```python
from build123d import *

# Parameters (mm, degrees)
SKETCH1_R           = 2.6
BOSS_EXTRUDE1_DEPTH = 20
BOSS_EXTRUDE2_DEPTH = 20
BOSS_EXTRUDE3_DEPTH = 180
CUT_EXTRUDE1_DEPTH  = 195.584574731


with BuildPart() as part:
    # Sketch1 → Boss-Extrude1 (new body)
    with BuildSketch(Plane(origin=(0, 0, 0), x_dir=(1, 0, 0), z_dir=(0, 1, 0))):
        with BuildLine():
            Line((10, 0), (-10, 0))
            ThreePointArc((-10, 0), (-2.947752983, 31.810630591), (16.887506811, 57.660444431))
            Line((16.887506811, 57.660444431), (29.743259005, 42.339555569))
            ThreePointArc((29.743259005, 42.339555569), (15.178402758, 23.358265357), (10, 0))
        make_face()
        with Locations(Location((0.770593323, 10, 0), (0, 0, 270))):
            Circle(SKETCH1_R, mode=Mode.SUBTRACT)
        with Locations(Location((6.115324888, 27.584447974, 0), (0, 0, 270))):
            Circle(SKETCH1_R, mode=Mode.SUBTRACT)
        with Locations(Location((16.150266317, 42.98181517, 0), (0, 0, 270))):
            Circle(SKETCH1_R, mode=Mode.SUBTRACT)
    extrude(amount=BOSS_EXTRUDE1_DEPTH)

    # Sketch2 → Boss-Extrude2 (add)
    with BuildSketch(Plane(origin=(0, 20, 0), x_dir=(1, 0, 0), z_dir=(0, 1, 0))):
        Polygon((16.887506811, 57.660444431), (29.743259005, 42.339555569), (34.416130108, 46.260559988), (21.560377914, 61.58144885), align=None)
    extrude(amount=-BOSS_EXTRUDE2_DEPTH)

    # Sketch4 → Cut-Extrude1 (cut, through all)
    with BuildSketch(Plane(origin=(0, 20, 0), x_dir=(1, 0, 0), z_dir=(0, 1, 0))):
        with BuildLine():
            Line((29.743259005, 42.339555569), (34.416130108, 46.260559988))
            Line((34.416130108, 46.260559988), (21.560377914, 61.58144885))
            Line((21.560377914, 61.58144885), (16.887506811, 57.660444431))
            ThreePointArc((16.887506811, 57.660444431), (-2.947752983, 31.810630591), (-10, 0))
            Line((-10, 0), (10, 0))
            ThreePointArc((10, 0), (15.178402758, 23.358265357), (29.743259005, 42.339555569))
        make_face()
    extrude(amount=-CUT_EXTRUDE1_DEPTH, mode=Mode.SUBTRACT)


with BuildPart() as body_2:
    # Sketch3 → Boss-Extrude3 (new body)
    with BuildSketch(Plane(origin=(0, 20, 0), x_dir=(1, 0, 0), z_dir=(0, 1, 0))):
        with BuildLine():
            Line((18.346439865, 65.411671066), (13.673568762, 61.490666647))
            ThreePointArc((13.673568762, 61.490666647), (-7.479291918, 33.9237219), (-15, 0))
            Line((-15, 0), (-10, 0))
            ThreePointArc((-10, 0), (-2.947752983, 31.810630591), (16.887506811, 57.660444431))
            Line((16.887506811, 57.660444431), (21.560377914, 61.58144885))
            Line((21.560377914, 61.58144885), (18.346439865, 65.411671066))
        make_face()
    extrude(amount=BOSS_EXTRUDE3_DEPTH)


solid = body_2.part
```
Geometry: final body of the model. Coordinates: model frame, mm. Round coordinates to 2 decimals unless told otherwise and drop trailing zeros. Write each loop counter-clockwise with the first axis right and the second up, starting at its lowest first coordinate (ties: lowest second). Pieces come first, ordered by that corner, then holes.
Item 1: Section query C-C (x = 3). Return loops of the section in (y, z).
Item 2: Pin query (flat end, axial travel): P1, Ø8, axis at y = 61, z = -15, coming from the +X side; P2, Ø5, axis at y = 153.5, z = -46.5, coming from the -X side; P3, Ø2, axis at y = 96, z = -34.5, coming from the -X side; P4, Ø8, axis at x = -7.5, z = -48, coming from the +Y side. Return the tip coordinate at first contact, or that it passes through.
Item 3: Section query B-B (z = -21). Return loops of the section in (x, y).
Item 4: Section query A-A (y = 188). Return loops of the section in (x, z).
Item 5: Material intervals for L1, parallel to X at y = 175.5, z = -26.5; L2, parallel to X at y = 53, z = -27; L3, parallel to Z at x = 10.5, y = 120, sorted ascending.
Completed:
1. outline: (20, -50.65) - (200, -50.65) - (200, -42.29) - (20, -42.29) - close
2. P1: stops at x = -7.56
2. P2: stops at x = -1.87
2. P3: stops at x = -7.68
2. P4: passes through
3. outline: (-12.2, 20) - (-7.01, 20) - (-7.01, 200) - (-12.2, 200) - close
4. outline: (-15, 0) arc R80.27 ccw to (13.67, -61.49) - (18.35, -65.41) - (21.56, -61.58) - (16.89, -57.66) arc R75.27 cw to (-10, 0) - close
5. L1: x = -10.5 to -5.18
5. L2: x = -10.32 to -4.99
5. L3: z = -58.68 to -51.63
